Model file for the job. Use its own axes, mm. Round coordinates to 2 decimals unless told otherwise and drop trailing zeros. Write each loop counter-clockwise with the first axis right and the second up, starting at its lowest first coordinate (ties: lowest second). Pieces come first, ordered by that corner, then holes. Notation, with made-up numbers: (7.5, -36.5) - (30.5, -36.5) arc R15 ccw to (30.5, -18.5) - close; hole circle Ø5 at (-37.75, -15.75). An arc over 180 degrees is marked (long way). One line per item, written item: value.
from build123d import *

# Parameters (mm, degrees)
SKETCH1_W           = 42
SKETCH1_H           = 24
BOSS_EXTRUDE1_DEPTH = 1
SKETCH2_R           = 1
CUT_EXTRUDE1_DEPTH  = 2
FILLET1_R           = 2


with BuildPart() as part:
    # Sketch1 → Boss-Extrude1 (new body)
    with BuildSketch(Plane(origin=(0, 0, 0), x_dir=(1, 0, 0), z_dir=(0, 1, 0))):
        Rectangle(SKETCH1_W, SKETCH1_H)
    extrude(amount=BOSS_EXTRUDE1_DEPTH)

    # Sketch2 → Cut-Extrude1 (cut, through all)
    with BuildSketch(Plane(origin=(0, 1, 0), x_dir=(1, 0, 0), z_dir=(0, 1, 0))):
        with Locations((-19, 10)):
            Circle(SKETCH2_R)
        with Locations((-19, -10)):
            Circle(SKETCH2_R)
        with Locations((19, -10)):
            Circle(SKETCH2_R)
        with Locations((19, 10)):
            Circle(SKETCH2_R)
    extrude(amount=-CUT_EXTRUDE1_DEPTH, mode=Mode.SUBTRACT)

    # Fillet1
    fillet1_edges = [part.edges().sort_by_distance(p)[0] for p in [
        (21, 0.5, 12),
        (-21, 0.5, 12),
        (-21, 0.5, -12),
        (21, 0.5, -12),
    ]]
    fillet(fillet1_edges, radius=FILLET1_R)


solid = part.part
1. Band-saw the part on A-A on y = 0.6. Write the cut outline in (x, z), plus the area to 3 significant figures.
Report:
outline: (-21, -10) arc R2 ccw to (-19, -12) - (19, -12) arc R2 ccw to (21, -10) - (21, 10) arc R2 ccw to (19, 12) - (-19, 12) arc R2 ccw to (-21, 10) - close; hole circle Ø2 at (-19, -10); hole circle Ø2 at (-19, 10); hole circle Ø2 at (19, -10); hole circle Ø2 at (19, 10)
area: 992 mm²
2. Wall check: probe 1 along X at (y, z) = (0.3, -10); probe 2 along Z at (x, y) = (19, 0.2). Give the ranges that are in metal, low to high. Write a range as [from, to].
Report:
probe 1: [-21, -20], [-18, 18], [20, 21]
probe 2: [-12, -11], [-9, 9], [11, 12]
3. Drop a flat-ended pin along its axis: pin 1 (2.5 mm diameter, centred on x = 19, z = 10, fed in from -Y). Give the stop position or say it passes through.
Report:
pin 1: y = 0
4. Mould opens along Z. For faces 1 (the face through (-0.3, 0.5, -12)), 2 (the face through (0, 1, 0)), 3 (the face through (-19.737, 0.507, -10.676)) say: released by +Z, released by -Z, zero draft, split by the parting line, or undercut.
Report:
face 1: released by -Z
face 2: zero draft
face 3: undercut
